Part model, mm, in its own coordinate system. A direction names the side the tool comes from. Coordinates: 2 decimals unless noted, no trailing zeros. Order: outer loops, then holes, each group sorted by start corner. A loop starts at its lowest first (then second) coordinate and runs counter-clockwise, first axis right, second up.
1) Pin check, flat tips, straight feed: pin 1 Ø3 at (x, z) = (-7.5, 3.5) entering from -Y; pin 2 Ø2.5 at (x, z) = (-17, 4.5) entering from -Y. Stop position of each tip, or through.
2) Cut at B-B (z = 2). List the corners of the cut face in (x, y).
3) Mould opens along X. For faces 1 (the flat face through (1.494, 16, 3)), 2 (the flat face through (-4.856, 25, 3)), 3 (the flat face through (-2, 9.338, 3)), 4 (the flat face through (-10, 28.388, 3)) say: +X half, -X half, draft (parallel to the pull), parting line (faces both ways), or undercut.
4) Cut at D-D (x = -23.5). List the corners of the cut face in (y, z), and give its area (3 significant figures).
5) Cut at C-C (y = -120). List the corners of the cut face in (x, z), and give its area (3 significant figures).
6) Cut at A-A (x = -1.5). List the corners of the cut face in (y, z).
7) Tool access for faces 5 (the flat face through (-14.381, 25, 3)), 6 (the flat face through (-2, 22.038, 3)), 7 (the flat face through (-4.856, -65, 3)): list every direction of +Z, -Z, +X, -X, +Y, -Y with a clear straight run to the whole face (end or side of a thin tool).
8) Wall check: L1, parallel to Y at x = -20, z = 1; L2, parallel to X at y = -78.5, z = 2.75; L3, parallel to Y at x = -16.5, z = 5.75. Give the ranges that are in metal, low to high.
```python
from build123d import *

# Parameters (mm, degrees)
F0_W     = 6.35
F0_H     = 6.35
F0_H_2   = 146.05
F0_W_2   = 4.7625
F1_DEPTH = 6.35


with BuildPart() as f1:
    # F0 (on Top) → F1 (new body)
    with BuildSketch(Plane.XY):
        Polygon((7.844118, -136.711765), (7.844118, 15.688235), (1.494118, 15.688235), (1.494118, 9.338235), (1.494118, -136.711765), align=None)
        with Locations((4.669118, 18.863235)):
            Rectangle(F0_W, F0_H)
        Polygon((1.494118, 22.038235), (7.844118, 22.038235), (7.844118, 28.388235), (-4.855882, 28.388235), (-4.855882, 22.038235), align=None)
        with Locations((-1.680882, -63.686765)):
            Rectangle(F0_W, F0_H_2)
        Polygon((-4.855882, 28.388235), (7.844118, 28.388235), (7.844118, 34.738235), (-30.255882, 34.738235), (-30.255882, 28.388235), (-19.143382, 28.388235), (-14.380882, 28.388235), align=None)
        with Locations((-16.762132, 25.213235)):
            Rectangle(F0_W_2, F0_H)
    extrude(amount=F1_DEPTH)


solid = f1.part
```
Geometry check:
1. pin 1: stops at y = 28.39
1. pin 2: stops at y = 22.04
2. outline: (-30.26, 28.39) - (-19.14, 28.39) - (-19.14, 22.04) - (-14.38, 22.04) - (-14.38, 28.39) - (-4.86, 28.39) - (-4.86, 22.04) - (1.49, 22.04) - (1.49, 9.34) - (-4.86, 9.34) - (-4.86, -136.71) - (7.84, -136.71) - (7.84, 34.74) - (-30.26, 34.74) - close
3. face 1: -X half
3. face 2: undercut
3. face 3: draft
3. face 4: undercut
4. outline: (28.39, 0) - (34.74, 0) - (34.74, 6.35) - (28.39, 6.35) - close
4. area: 40.3 mm2
5. outline: (-4.86, 0) - (7.84, 0) - (7.84, 6.35) - (-4.86, 6.35) - close
5. area: 80.6 mm2
6. outline: (-136.71, 0) - (9.34, 0) - (9.34, 6.35) - (-136.71, 6.35) - close; (22.04, 0) - (34.74, 0) - (34.74, 6.35) - (22.04, 6.35) - close
7. face 5: +Z, -Z, -Y
7. face 6: +Z, -Z, -X
7. face 7: +Z, -Z, -X, -Y
8. L1: y = 28.39 to 34.74
8. L2: x = -4.86 to 7.84
8. L3: y = 22.04 to 34.74
